from build123d import *

# Parameters (mm, degrees)
SKETCH1_W           = 22.722789772
SKETCH1_H           = 28
SKETCH1_R           = 1.65
BOSS_EXTRUDE1_DEPTH = 3.175
SKETCH2_W           = 3.175
SKETCH2_H           = 28
BOSS_EXTRUDE2_DEPTH = 40
FILLET1_R           = 10
SKETCH3_R           = 1.15
CUT_EXTRUDE1_DEPTH  = 3.175


with BuildPart() as part:
    # Sketch1 → Boss-Extrude1 (new body)
    with BuildSketch(Plane(origin=(0, 0, 0), x_dir=(1, 0, 0), z_dir=(0, 1, 0))):
        Rectangle(SKETCH1_W, SKETCH1_H)
        with Locations((8.361394886, 10.30327082)):
            Circle(SKETCH1_R, mode=Mode.SUBTRACT)
        with Locations((8.361394886, -10.30327082)):
            Circle(SKETCH1_R, mode=Mode.SUBTRACT)
    extrude(amount=BOSS_EXTRUDE1_DEPTH)

    # Sketch2 → Boss-Extrude2 (add)
    with BuildSketch(Plane(origin=(0, 3.175, 0), x_dir=(1, 0, 0), z_dir=(0, 1, 0))):
        with Locations((-9.773894886, 0)):
            Rectangle(SKETCH2_W, SKETCH2_H)
    extrude(amount=BOSS_EXTRUDE2_DEPTH)

    # Fillet1
    fillet1_edges = [part.edges().sort_by_distance(p)[0] for p in [
        (-8.186394886, 3.175, 0),
        (-11.361394886, 0, 0),
    ]]
    fillet(fillet1_edges, radius=FILLET1_R)

    # Sketch3 → Cut-Extrude1 (cut)
    with BuildSketch(Plane.ZY.offset(11.361394886)):
        with Locations((10.5, 40.305754395)):
            Circle(SKETCH3_R)
        with Locations((10.5, 27.805754395)):
            Circle(SKETCH3_R)
        with Locations((-10.5, 40.305754395)):
            Circle(SKETCH3_R)
        with Locations((-10.5, 27.805754395)):
            Circle(SKETCH3_R)
    extrude(amount=-CUT_EXTRUDE1_DEPTH, mode=Mode.SUBTRACT)


solid = part.part
Input: part model. Units: mm. Frame: model coordinates. A direction names the side the tool comes from. Coordinates: 2 decimals unless noted, no trailing zeros. Loops run counter-clockwise (first coordinate to the right, second up) from the corner with the lowest first, then second, coordinate; pieces in that order, holes last.
(1) Section D-D on y = 36.5. Return the cut outline in (x, z).
(2) Material intervals for probe 1 along Y at (x, z) = (-8.8, -10.5) (3 decimals); probe 2 along Y at (x, z) = (-10.1, -10.5) (3 decimals); probe 3 along X at (y, z) = (34, -4), sorted ascending.
(3) Pull-direction query (Z, two-part tool) for faces 1 (the face through (-9.796, 39.183, -10.749)), 2 (the face through (-5.18, 6.03, -0.2)), 3 (the face through (-9.796, 28.775, 11.118)), 4 (the face through (-8.5, 15.1, 14)); classes: released by +Z, released by -Z, zero draft, split by the parting line, or undercut.
(4) First-contact query: pin 1 Ø4.5 at (x, z) = (8.36, -10.3) entering from -Y; pin 2 Ø10 at (x, z) = (5.5, 4.5) entering from +Y; pin 3 Ø2 at (y, z) = (8.5, 10) entering from +X; pin 4 Ø2.5 at (y, z) = (40.31, -10.5) entering from +X. Flat tips, straight axial feed; report the tip coordinate or a pass-through.
(5) Set-up query: faces 5 (the face through (-8.186, 28, 0)), 6 (the face through (7.052, 1.565, 11.307)). Return all of +Z, -Z, +X, -X, +Y, -Y with unobstructed straight access to the full face (end or side cutting, diameter ignored); none if empty.
(6) Section B-B on y = 28.5. Return the cut outline in (x, z).
(7) Section A-A on z = -7.25. Return the cut outline in (x, y) (3 decimals).
(8) Section C-C on x = 8. Return the cut outline in (y, z) (3 decimals), then the cut area to 3 significant figures.
Data:
1. outline: (-11.36, -14) - (-8.19, -14) - (-8.19, 14) - (-11.36, 14) - close
2. probe 1: y = 3.317 to 26.656, 28.956 to 39.156, 41.456 to 43.175
2. probe 2: y = 5.138 to 26.656, 28.956 to 39.156, 41.456 to 43.175
2. probe 3: x = -11.36 to -8.19
3. face 1: undercut
3. face 2: zero draft
3. face 3: undercut
3. face 4: released by +Z
4. pin 1: stops at y = 0
4. pin 2: stops at y = 3.26
4. pin 3: stops at x = -6.42
4. pin 4: stops at x = -8.19
5. face 5: +Z, -Z, +X, +Y
5. face 6: +Y, -Y
6. outline: (-11.36, -14) - (-8.19, -14) - (-8.19, -11.42) - (-11.36, -11.42) - close; (-11.36, -9.58) - (-8.19, -9.58) - (-8.19, 9.58) - (-11.36, 9.58) - close; (-11.36, 11.42) - (-8.19, 11.42) - (-8.19, 14) - (-11.36, 14) - close
7. outline: (-11.361, 10) arc R10 ccw to (-1.361, 0) - (11.361, 0) - (11.361, 3.175) - (1.814, 3.175) arc R10 cw to (-8.186, 13.175) - (-8.186, 43.175) - (-11.361, 43.175) - close
8. outline: (0, -14) - (3.175, -14) - (3.175, -11.913) - (0, -11.913) - close; (0, -8.693) - (3.175, -8.693) - (3.175, 8.693) - (0, 8.693) - close; (0, 11.913) - (3.175, 11.913) - (3.175, 14) - (0, 14) - close
8. area: 68.5 mm2
